The model under review builds one solid part; all positions refer to its coordinate system, in mm. A direction names the side the tool comes from. Coordinates: 2 decimals unless noted, no trailing zeros. Write each loop counter-clockwise with the first axis right and the second up, starting at its lowest first coordinate (ties: lowest second). Pieces come first, ordered by that corner, then holes.
1) Add section C-C, the plane x = 2.04. State the section outline as (y, z) points, then the cut area to 3 significant figures.
2) For P1, Ø0.5, axis at x = 6, z = 3, coming from the -Y side; P2, Ø0.8, axis at x = 10, z = 3, coming from the +Y side; P3, Ø1.2, axis at x = 4.5, y = 4, coming from the +Z side, all flat-tipped, find the tip position at first contact; note any pin that passes through.
3) Add section B-B, the plane z = 2.9. Give the number of separate pieces and of enclosed holes in the cut face, then the cut area to 3 significant figures.
4) Add section A-A, the plane y = 6. State the section outline as (x, z) points, then the cut area to 3 significant figures.
5) Machinability: for faces 5 (the flat face through (9.7, 1, 2.1)), 6 (the flat face through (6, 2, 4)), 7 (the flat face through (2.54, 0.27, 2.07)), which of the approach directions +Z, -Z, +X, -X, +Y, -Y give a long, thin tool a straight path to every point of the face, cutting with its end or side? Answer none if there is none.
6) Add section D-D, the plane z = -0.25. State the section outline as (x, y) points, then the cut area to 3 significant figures.
7) For line 1 (X direction, y = 5, z = 3.25); line 2 (Z direction, x = 10.25, y = 3.5); line 3 (X direction, y = 2.5, z = 3), list the stretches that pass through material, from the lowest coordinate up.
8) Mouldability with a two-part tool opening along Z and no side actions: class faces 1 (the flat face through (6, 2, 7.2)), 2 (the cylindrical face through (10, 6.1, 0.6)), 3 (the cylindrical face through (2.1, 6.1, 0.6)), 4 (the flat face through (6, 0, 5)) as released by +Z, released by -Z, zero draft, split by the parting line, or undercut.
from build123d import *

# Parameters (mm, degrees)
SKETCH_1_W             = 12
SKETCH_1_H             = 10
EXTRUDE_1_DEPTH        = 7.2
SKETCH_2_W             = 1.17709233
SKETCH_2_H             = 4
CUT_EXTRUDE_1_DEPTH    = 18.2
CUT_EXTRUDE_2_DEPTH    = 18.2
SKETCH_4_W             = 1
SKETCH_4_H             = 4.2
CUT_EXTRUDE_3_DEPTH    = 1
PATTERN_LINEAR_1_COUNT = 2
PATTERN_LINEAR_1_PITCH = 3.96
PATTERN_LINEAR_2_COUNT = 2
PATTERN_LINEAR_2_PITCH = 3.96
SKETCH_5_R             = 0.4
EXTRUDE_3_DEPTH        = 5.8
PATTERN_LINEAR_3_COUNT = 3
PATTERN_LINEAR_3_PITCH = 3.96
CUT_EXTRUDE_4_DEPTH    = 8
SKETCH_7_R             = 0.5
EXTRUDE_4_DEPTH        = 6


with BuildPart() as part:
    # 草图1 → 凸台-拉伸1 (new body)
    with BuildSketch(Plane.XY):
        with Locations((6, 5)):
            Rectangle(SKETCH_1_W, SKETCH_1_H)
    extrude(amount=EXTRUDE_1_DEPTH)

    # 草图2 → 切除-拉伸1 (cut, through all)
    with BuildSketch(Plane(origin=(12, 0, 0), x_dir=(0, 0, -1), z_dir=(1, 0, 0))):
        with Locations((-7.588546165, 5)):
            Rectangle(SKETCH_2_W, SKETCH_2_H)
    extrude(amount=-CUT_EXTRUDE_1_DEPTH, mode=Mode.SUBTRACT)

    # 草图3 → 切除-拉伸2 (cut, through all)
    with BuildSketch(Plane(origin=(12, 0, 0), x_dir=(0, 0, -1), z_dir=(1, 0, 0))):
        Polygon((-7, 10), (-7.2, 8.5), (-7.2, 10), align=None)
    extrude(amount=-CUT_EXTRUDE_2_DEPTH, mode=Mode.SUBTRACT)

    # 草图4 → 切除-拉伸3 (cut)
    with BuildSketch(Plane.XZ):
        with Locations((6, 2.1)):
            Rectangle(SKETCH_4_W, SKETCH_4_H)
    cut_extrude_3 = extrude(amount=-CUT_EXTRUDE_3_DEPTH, mode=Mode.SUBTRACT)

    # 阵列(线性)1: 切除-拉伸3 ×2
    with Locations(*[(i * PATTERN_LINEAR_1_PITCH, 0, 0) for i in range(1, PATTERN_LINEAR_1_COUNT)]):
        add(cut_extrude_3, mode=Mode.SUBTRACT)

    # 阵列(线性)2: 切除-拉伸3 ×2
    with Locations(*[(-i * PATTERN_LINEAR_2_PITCH, 0, 0) for i in range(1, PATTERN_LINEAR_2_COUNT)]):
        add(cut_extrude_3, mode=Mode.SUBTRACT)

    # 草图5 → 凸台-拉伸3 (add)
    with BuildSketch(Plane(origin=(0, 0, 4.2), x_dir=(-1, 0, 0), z_dir=(0, 0, -1))):
        with Locations(Location((-2.04, 0.5, 0), (0, 0, 180))):
            Circle(SKETCH_5_R)
    extrude_3 = extrude(amount=EXTRUDE_3_DEPTH)

    # 阵列(线性)3: 凸台-拉伸3 ×3
    with Locations(*[(i * PATTERN_LINEAR_3_PITCH, 0, 0) for i in range(1, PATTERN_LINEAR_3_COUNT)]):
        add(extrude_3)

    # 草图6 → 切除-拉伸4 (cut)
    with BuildSketch(Plane(origin=(0, 10, 0), x_dir=(1, 0, 0), z_dir=(0, 1, 0))):
        with BuildLine():
            Line((0, -5.8), (12, -5.8))
            Line((12, -5.8), (12, -4.26427845))
            Line((12, -4.26427845), (12, -1.4))
            Line((12, -1.4), (11.748854382, -1.4))
            ThreePointArc((11.748854382, -1.4), (9.96, -0.6), (8.171145618, -1.4))
            Line((8.171145618, -1.4), (7.788854382, -1.4))
            ThreePointArc((7.788854382, -1.4), (6, -0.6), (4.211145618, -1.4))
            Line((4.211145618, -1.4), (3.828854382, -1.4))
            ThreePointArc((3.828854382, -1.4), (2.04, -0.6), (0.251145618, -1.4))
            Line((0.251145618, -1.4), (0, -1.4))
            Line((0, -1.4), (0, -5.8))
        make_face()
    extrude(amount=-CUT_EXTRUDE_4_DEPTH, mode=Mode.SUBTRACT)

    # 草图7 → 凸台-拉伸4 (add)
    with BuildSketch(Plane(origin=(0, 2, 0), x_dir=(-1, 0, 0), z_dir=(0, 1, 0))):
        with Locations(Location((-6, 2.9, 0), (0, 0, 90))):
            Circle(SKETCH_7_R)
        with Locations(Location((-9.96, 2.9, 0), (0, 0, 90))):
            Circle(SKETCH_7_R)
        with Locations(Location((-2.04, 2.9, 0), (0, 0, 90))):
            Circle(SKETCH_7_R)
    extrude(amount=EXTRUDE_4_DEPTH)


solid = part.part
Geometry results:
1. outline: (0, 4.2) - (0.1, 4.2) - (0.1, -1.6) - (0.9, -1.6) - (0.9, 4.2) - (1, 4.2) - (1, 0) - (10, 0) - (10, 0.6) - (2, 0.6) - (2, 2.4) - (8, 2.4) - (8, 3.4) - (2, 3.4) - (2, 5.8) - (10, 5.8) - (10, 7) - (8.5, 7.2) - (7, 7.2) - (7, 7) - (3, 7) - (3, 7.2) - (0, 7.2) - close
1. area: 35.9 mm2
2. P1: stops at y = 0.1
2. P2: stops at y = 8
2. P3: stops at z = 7
3. separate pieces: 4
3. enclosed holes: 0
3. area: 40.5 mm2
4. outline: (0, 0) - (12, 0) - (12, 1.4) - (11.75, 1.4) arc R2.4 cw to (8.17, 1.4) - (7.79, 1.4) arc R2.4 cw to (4.21, 1.4) - (3.83, 1.4) arc R2.4 cw to (0.25, 1.4) - (0, 1.4) - close; (0, 5.8) - (12, 5.8) - (12, 7) - (0, 7) - close; circle Ø1 at (2.04, 2.9); circle Ø1 at (6, 2.9); circle Ø1 at (9.96, 2.9)
4. area: 27.6 mm2
5. face 5: -Z
5. face 6: +Y
5. face 7: -Z, -Y
6. outline: circle Ø0.8 at (2.04, 0.5); circle Ø0.8 at (6, 0.5); circle Ø0.8 at (9.96, 0.5)
6. area: 1.51 mm2
7. line 1: x = 1.68 to 2.4, 5.64 to 6.36, 9.6 to 10.32
7. line 2: z = 0 to 0.62, 2.49 to 3.31, 5.8 to 7
7. line 3: x = 1.55 to 2.53, 5.51 to 6.49, 9.47 to 10.45
8. face 1: released by +Z
8. face 2: undercut
8. face 3: undercut
8. face 4: zero draft
